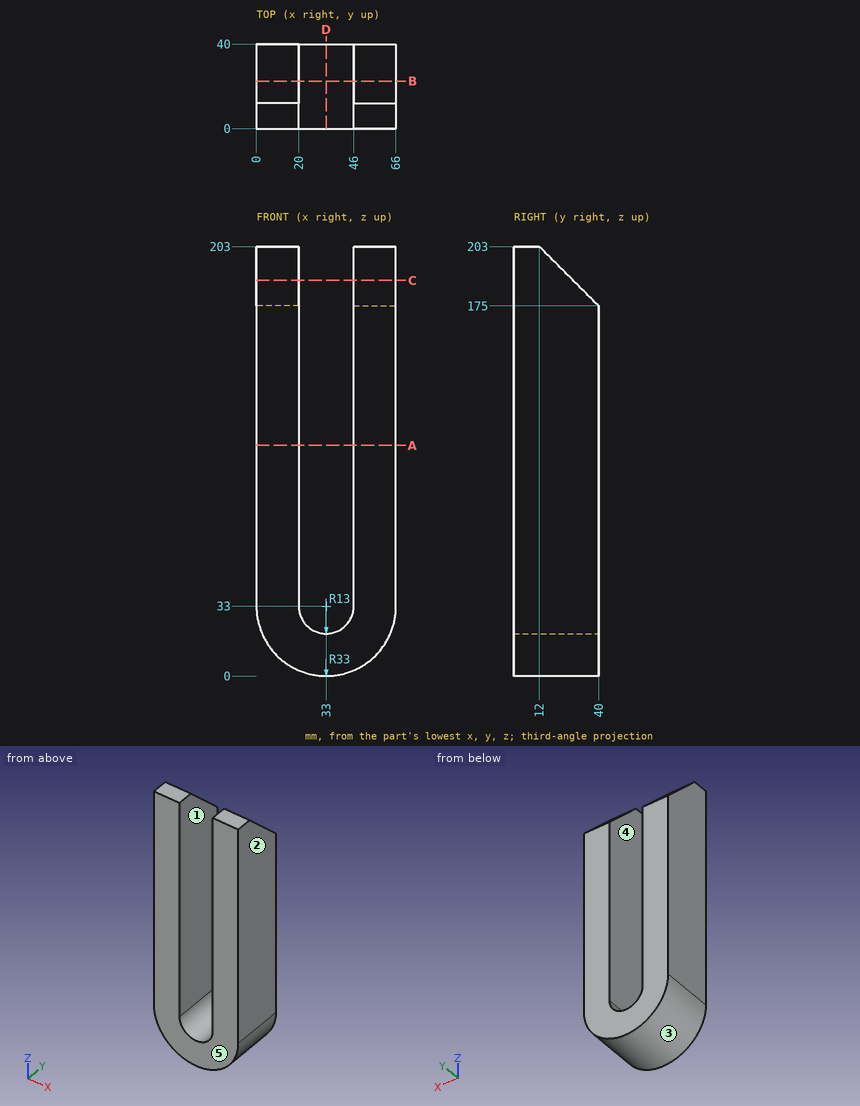
Source: three-view drawing plus pictorial views. Frame: mm from the lowest corner of the part. A direction names the side the tool comes from. Coordinates: 2 decimals unless noted, no trailing zeros. Order: outer loops, then holes, each group sorted by start corner. A loop starts at its lowest first (then second) coordinate and runs counter-clockwise, first axis right, second up.
Item 1: Material intervals for line 1 (X direction, y = 31, z = 177.5); line 2 (X direction, y = 17, z = 21.5); line 3 (Z direction, x = 33, y = 14), sorted ascending.
Output values:
line 1: x = 0 to 20, 46 to 66
line 2: x = 2.07 to 26.94, 39.06 to 63.93
line 3: z = 0 to 20
Item 2: Set-up query: the marked faces 1 and 2. Return all of +Z, -Z, +X, -X, +Y, -Y with unobstructed straight access to the full face (end or side cutting, diameter ignored); none if empty.
Output values:
face 1: +Z, +Y, -Y
face 2: +Z, -Z, +X, +Y, -Y
Item 3: Cut plane D-D (x = 33). Return loops of the section in (y, z), plus the area to 3 significant figures.
Output values:
outline: (0, 0) - (40, 0) - (40, 20) - (0, 20) - close
area: 800 mm2
Item 4: First-contact query: P1, Ø12, axis at y = 25, z = 140, coming from the -X side; P2, Ø2, axis at x = 49, y = 13.5, coming from the +Z side; P3, Ø4, axis at x = 57.5, y = 25.5, coming from the +Z side; P4, Ø6, axis at x = 21, y = 18.5, coming from the -Z side. Flat tips, straight axial feed; report the tip coordinate or a pass-through.
Output values:
P1: stops at x = 0
P2: stops at z = 202.5
P3: stops at z = 191.5
P4: stops at z = 1.25
Item 5: Cut plane A-A (z = 109). Return loops of the section in (x, y).
Output values:
outline: (0, 0) - (20, 0) - (20, 40) - (0, 40) - close; (46, 0) - (66, 0) - (66, 40) - (46, 40) - close
Item 6: Pull-direction query (X, two-part tool) for the marked faces 3, 4 and 5; classes: pulls with the +X half, pulls with the -X half, needs draft (parallel to the pull), parting line crosses it, or undercut.
Output values:
face 3: parting line crosses it
face 4: undercut
face 5: needs draft
Item 7: Cut plane C-C (z = 187). Return loops of the section in (x, y).
Output values:
outline: (0, 0) - (20, 0) - (20, 28) - (0, 28) - close; (46, 0) - (66, 0) - (66, 28) - (46, 28) - close
Item 8: Cut plane B-B (y = 22.5). Return loops of the section in (x, z).
Output values:
outline: (0, 33) arc R33 ccw to (66, 33) - (66, 192.5) - (46, 192.5) - (46, 33) arc R13 cw to (20, 33) - (20, 192.5) - (0, 192.5) - close
